```python
from build123d import *

# Parameters (mm, degrees)
SKETCH1_R           = 3.81
SKETCH1_R_2         = 1.651
BOSS_EXTRUDE1_DEPTH = 6.35
FILLET2_R           = 5.08
SKETCH3_R           = 1.5875
CUT_EXTRUDE1_DEPTH  = 6.35
CUT_EXTRUDE2_DEPTH  = 6.35


with BuildPart() as part:
    # Sketch1 → Boss-Extrude1 (new body)
    with BuildSketch(Plane.XY):
        with BuildLine():
            Line((0, 0), (101.6, 0))
            Line((101.6, 0), (79.43330905, 22.16669095))
            Line((79.43330905, 22.16669095), (98.16062093, 25.658150496))
            ThreePointArc((98.16062093, 25.658150496), (110.542778436, 42.04253584), (95.367453293, 55.88))
            Line((95.367453293, 55.88), (0, 38.1))
            Line((0, 38.1), (0, 25.4))
            Line((0, 25.4), (-6.35, 25.4))
            Line((-6.35, 25.4), (-6.35, 12.7))
            Line((-6.35, 12.7), (0, 12.7))
            Line((0, 12.7), (0, 0))
        make_face()
        with Locations((95.367453293, 40.64)):
            Circle(SKETCH1_R, mode=Mode.SUBTRACT)
        with Locations((25.817011896, 25.817011896)):
            Circle(SKETCH1_R_2, mode=Mode.SUBTRACT)
        with Locations((25.817011896, 12.282988104)):
            Circle(SKETCH1_R_2, mode=Mode.SUBTRACT)
        with Locations((12.282988104, 12.282988104)):
            Circle(SKETCH1_R_2, mode=Mode.SUBTRACT)
        with Locations((12.282988104, 25.817011896)):
            Circle(SKETCH1_R_2, mode=Mode.SUBTRACT)
    extrude(amount=BOSS_EXTRUDE1_DEPTH)

    # Fillet2
    fillet2_edges = [part.edges().sort_by_distance(p)[0] for p in [
        (79.43330905, 22.16669095, 3.175),
    ]]
    fillet(fillet2_edges, radius=FILLET2_R)

    # Sketch3 → Cut-Extrude1 (cut)
    with BuildSketch(Plane.ZY):
        with Locations(Location((3.175, 31.75, 0), (0, 0, 270))):
            Circle(SKETCH3_R)
        with Locations(Location((3.175, 6.35, 0), (0, 0, 270))):
            Circle(SKETCH3_R)
    extrude(amount=-CUT_EXTRUDE1_DEPTH, mode=Mode.SUBTRACT)

    # Sketch6 → Cut-Extrude2 (cut)
    with BuildSketch(Plane.XY.offset(6.35)):
        with BuildLine():
            Line((50.8, 0), (76.2, 0))
            ThreePointArc((76.2, 0), (63.5, 12.7), (50.8, 0))
        make_face()
    extrude(amount=-CUT_EXTRUDE2_DEPTH, mode=Mode.SUBTRACT)


solid = part.part
```
Model file for the job. Use its own axes, mm. A direction names the side the tool comes from. Round coordinates to 2 decimals unless told otherwise and drop trailing zeros. Loops run counter-clockwise (first coordinate to the right, second up) from the corner with the lowest first, then second, coordinate; pieces in that order, holes last. Notation, with made-up numbers: M 56.25,88.25 L 62.25,88.25 A23 ccw 62.25,106.25 Z; hole C 8.5,-5 d4. An arc over 180 degrees is marked long. Put each result on its own line as item: value. Start each with the question number.
Item 1: Drop flat-ended pins along their axis: P1, Ø4, axis at x = 20, y = 24, coming from the -Z side; P2, Ø1, axis at y = 36.5, z = 2.5, coming from the -X side; P3, Ø3, axis at x = -2.5, z = 3.5, coming from the -Y side; P4, Ø1.9, axis at y = 6.35, z = 3.175, coming from the -X side. Give the stop position or say it passes through.
Item 2: Cut at A-A (y = 40.64). List the corners of the cut face in (x, z).
Item 3: Drill centre lines: line 1 along Y through (x, z) = (96, 6.25); line 2 along Z through (x, y) = (5, 6); line 3 along Y through (x, z) = (89, 4). Where is each one in solid material? Low to high.
Item 4: Cut at C-C (y = 6.35). List the corners of the cut face in (x, z), then the cut area to 3 significant figures.
Item 5: Cut at D-D (x = 63.5). List the corners of the cut face in (y, z), then the cut area to 3 significant figures.
Item 6: 3-axis set-ups, long thin cutter, end or side, ignore diameter. For faces 1 (the face through (0, 33, 5)), 2 (the face through (94, 7.6, 3.1)), 3 (the face through (0, 8, 4)), 4 (the face through (3.131, 5.497, 4.514)), 5 (the face through (51, 28, 6.35)): which of +Z, -Z, +X, -X, +Y, -Y reach the whole face in a straight line?
Item 7: Cut at B-B (y = 31.75). List the corners of the cut face in (x, z).
Item 8: Mould opens along Z. For faces 6 (the face through (-3, 12.7, 3)), 7 (the face through (51, 28, 0)), 8 (the face through (3.131, 30.236, 3.652)), 9 (the face through (6.35, 32, 3)) say: released by +Z, released by -Z, zero draft, split by the parting line, or undercut.
Answer block:
1. P1: z = 0
1. P2: x = 0
1. P3: y = 12.7
1. P4: x = 6.35
2. outline: M 13.62,0 L 91.56,0 L 91.56,6.35 L 13.62,6.35 Z; M 99.18,0 L 110.61,0 L 110.61,6.35 L 99.18,6.35 Z
3. line 1: 0 to 5.6, 25.26 to 36.88, 44.4 to 55.87
3. line 2: 0 to 1.63, 4.72 to 6.35
3. line 3: 0 to 12.6, 23.95 to 54.69
4. outline: M 0,0 L 52.5,0 L 52.5,6.35 L 0,6.35 L 0,4.76 L 6.35,4.76 L 6.35,1.59 L 0,1.59 Z; M 74.5,0 L 95.25,0 L 95.25,6.35 L 74.5,6.35 Z
4. area: 445 mm2
5. outline: M 12.7,0 L 49.94,0 L 49.94,6.35 L 12.7,6.35 Z
5. area: 236 mm2
6. face 1: +Z, -Z, -X, +Y
6. face 2: +Z, -Z, +X
6. face 3: +Z, -Z, -X, -Y
6. face 4: -X
6. face 5: +Z, +X, -X, +Y, -Y
7. outline: M 0,0 L 107.75,0 L 107.75,6.35 L 0,6.35 L 0,4.76 L 6.35,4.76 L 6.35,1.59 L 0,1.59 Z
8. face 6: zero draft
8. face 7: released by -Z
8. face 8: undercut
8. face 9: undercut
